```python
from build123d import *

# Parameters (mm, degrees)
F0_W     = 214.5938575268
F0_H     = 46.5465178713
F1_DEPTH = 25.4


with BuildPart() as f1:
    # F0 (on Front) → F1 (new body)
    with BuildSketch(Plane.XZ):
        with Locations((39.4191890955, 25.6276843138)):
            Rectangle(F0_W, F0_H)
        Polygon((-39.0857293959, 9.3650380149), (-58.7409636363, 9.3650380149), (-58.7409636363, 44.6240742319), (-54.6432292894, 44.6240742319), (-54.6432292894, 13.0769216701), (-39.0857293959, 13.0769216701), align=None, mode=Mode.SUBTRACT)
        Polygon((-6.697422326, 9.3650380149), (-10.9417799358, 9.3650380149), (-15.3327608085, 20.5778591187), (-29.4626131423, 20.5778591187), (-33.7995749182, 9.3650380149), (-37.951328362, 9.3650380149), (-24.0144013741, 44.7706974947), (-20.5648961894, 44.7706974947), align=None, mode=Mode.SUBTRACT)
        with BuildLine():
            Line((25.6908847439, 44.6240742319), (25.6908847439, 9.3650380149))
            Line((25.6908847439, 9.3650380149), (21.0143743593, 9.3650380149))
            Line((21.0143743593, 9.3650380149), (1.7449908106, 38.9520690624))
            Line((1.7449908106, 38.9520690624), (1.5520654647, 38.9520690624))
            add(Edge.make_bspline(
                [(1.5520654647, 38.9520690624), (1.9379161565, 33.743084723), (1.9379161565, 29.4061229472)],
                knots=[0, 0, 0, 1, 1, 1], degree=2))
            Line((1.9379161565, 29.4061229472), (1.9379161565, 9.3650380149))
            Line((1.9379161565, 9.3650380149), (-1.851137637, 9.3650380149))
            Line((-1.851137637, 9.3650380149), (-1.851137637, 44.6240742319))
            Line((-1.851137637, 44.6240742319), (2.7790706647, 44.6240742319))
            Line((2.7790706647, 44.6240742319), (22.0021521303, 15.152798392))
            Line((22.0021521303, 15.152798392), (22.1950774762, 15.152798392))
            add(Edge.make_bspline(
                [(22.1950774762, 15.152798392), (22.1487753932, 15.8010275542), (21.9790010888, 19.3354198911)],
                knots=[0, 0, 0, 1, 1, 1], degree=2))
            add(Edge.make_bspline(
                [(21.9790010888, 19.3354198911), (21.8092267844, 22.869812228), (21.8555288674, 24.3900639537)],
                knots=[0, 0, 0, 1, 1, 1], degree=2))
            Line((21.8555288674, 24.3900639537), (21.8555288674, 44.6240742319))
            Line((21.8555288674, 44.6240742319), (25.6908847439, 44.6240742319))
        make_face(mode=Mode.SUBTRACT)
        with BuildLine():
            add(Edge.make_bspline(
                [(58.9705069119, 40.0671775617), (63.5274035821, 35.5102808915), (63.5274035821, 27.3302462253)],
                knots=[0, 0, 0, 1, 1, 1], degree=2))
            add(Edge.make_bspline(
                [(63.5274035821, 27.3302462253), (63.5274035821, 18.6023035767), (58.7891570867, 13.9836707958)],
                knots=[0, 0, 0, 1, 1, 1], degree=2))
            add(Edge.make_bspline(
                [(58.7891570867, 13.9836707958), (54.0509105914, 9.3650380149), (45.1531936384, 9.3650380149)],
                knots=[0, 0, 0, 1, 1, 1], degree=2))
            Line((45.1531936384, 9.3650380149), (35.383454122, 9.3650380149))
            Line((35.383454122, 9.3650380149), (35.383454122, 44.6240742319))
            Line((35.383454122, 44.6240742319), (46.1872734925, 44.6240742319))
            add(Edge.make_bspline(
                [(46.1872734925, 44.6240742319), (54.4136102417, 44.6240742319), (58.9705069119, 40.0671775617)],
                knots=[0, 0, 0, 1, 1, 1], degree=2))
        make_face(mode=Mode.SUBTRACT)
        with BuildLine():
            add(Edge.make_bspline(
                [(97.7292089034, 40.3565655805), (101.9967175548, 35.533431933), (101.9967175548, 27.0447167133)],
                knots=[0, 0, 0, 1, 1, 1], degree=2))
            add(Edge.make_bspline(
                [(101.9967175548, 27.0447167133), (101.9967175548, 18.5791525352), (97.7137748758, 13.7290093392)],
                knots=[0, 0, 0, 1, 1, 1], degree=2))
            add(Edge.make_bspline(
                [(97.7137748758, 13.7290093392), (93.4308321967, 8.8788661433), (85.8141395406, 8.8788661433)],
                knots=[0, 0, 0, 1, 1, 1], degree=2))
            add(Edge.make_bspline(
                [(85.8141395406, 8.8788661433), (78.02767258, 8.8788661433), (73.7948904909, 13.644122187)],
                knots=[0, 0, 0, 1, 1, 1], degree=2))
            add(Edge.make_bspline(
                [(73.7948904909, 13.644122187), (69.5621084018, 18.4093782308), (69.5621084018, 27.0910187964)],
                knots=[0, 0, 0, 1, 1, 1], degree=2))
            add(Edge.make_bspline(
                [(69.5621084018, 27.0910187964), (69.5621084018, 35.7032062374), (73.8064660117, 40.4414527327)],
                knots=[0, 0, 0, 1, 1, 1], degree=2))
            add(Edge.make_bspline(
                [(73.8064660117, 40.4414527327), (78.0508236215, 45.1796992281), (85.8604416236, 45.1796992281)],
                knots=[0, 0, 0, 1, 1, 1], degree=2))
            add(Edge.make_bspline(
                [(85.8604416236, 45.1796992281), (93.4617002521, 45.1796992281), (97.7292089034, 40.3565655805)],
                knots=[0, 0, 0, 1, 1, 1], degree=2))
        make_face(mode=Mode.SUBTRACT)
        with BuildLine():
            Line((137.3946600207, 44.6240742319), (137.3946600207, 9.3650380149))
            Line((137.3946600207, 9.3650380149), (132.7181496361, 9.3650380149))
            Line((132.7181496361, 9.3650380149), (113.4487660875, 38.9520690624))
            Line((113.4487660875, 38.9520690624), (113.2558407416, 38.9520690624))
            add(Edge.make_bspline(
                [(113.2558407416, 38.9520690624), (113.6416914334, 33.743084723), (113.6416914334, 29.4061229472)],
                knots=[0, 0, 0, 1, 1, 1], degree=2))
            Line((113.6416914334, 29.4061229472), (113.6416914334, 9.3650380149))
            Line((113.6416914334, 9.3650380149), (109.8526376399, 9.3650380149))
            Line((109.8526376399, 9.3650380149), (109.8526376399, 44.6240742319))
            Line((109.8526376399, 44.6240742319), (114.4828459415, 44.6240742319))
            Line((114.4828459415, 44.6240742319), (133.7059274071, 15.152798392))
            Line((133.7059274071, 15.152798392), (133.898852753, 15.152798392))
            add(Edge.make_bspline(
                [(133.898852753, 15.152798392), (133.85255067, 15.8010275542), (133.6827763656, 19.3354198911)],
                knots=[0, 0, 0, 1, 1, 1], degree=2))
            add(Edge.make_bspline(
                [(133.6827763656, 19.3354198911), (133.5130020612, 22.869812228), (133.5593041442, 24.3900639537)],
                knots=[0, 0, 0, 1, 1, 1], degree=2))
            Line((133.5593041442, 24.3900639537), (133.5593041442, 44.6240742319))
            Line((133.5593041442, 44.6240742319), (137.3946600207, 44.6240742319))
        make_face(mode=Mode.SUBTRACT)
    extrude(amount=F1_DEPTH)


solid = f1.part
```
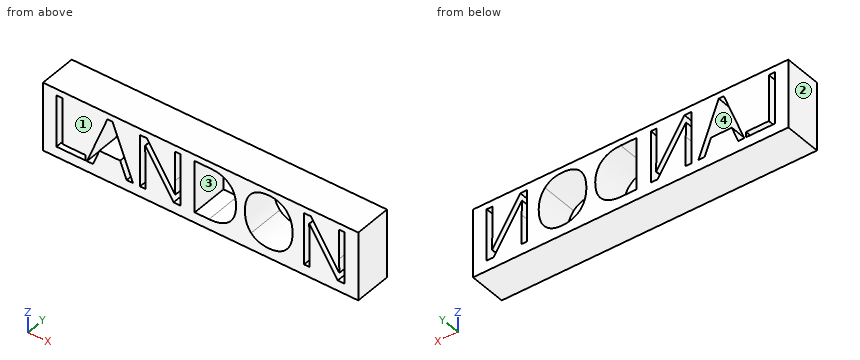
The listing builds one solid part. Answer for the finished solid, in the listing's coordinates (mm). Face numbers are marked on the shaded views. Give positions to 0.01 mm unless a question says otherwise; leave off trailing zeros. Order: outer loops, then holes, each group sorted by start corner. A loop starts at its lowest first (then second) coordinate and runs counter-clockwise, first axis right, second up. Notation, with made-up numbers: (0, 63) -> (20, 63) arc R28 cw to (20, 90) -> close; hole circle Ø9 at (4, -9.5). An arc over 180 degrees is marked (long way). Write each question's results on one line, items separated by ' | '.
Q1. The part is cut by section A-A, the plane x = 7.5. Give the vertices of the cut face in (y, z).
Checked values:
outline: (-25.4, 2.35) -> (0, 2.35) -> (0, 30.12) -> (-25.4, 30.12) -> close; (-25.4, 37.39) -> (0, 37.39) -> (0, 48.9) -> (-25.4, 48.9) -> close
Q2. The part is cut by section B-B, the plane y = -7.75. State how many separate pieces and enclosed holes the cut face has, and give its area (3 significant figures).
Checked values:
separate pieces: 1 | enclosed holes: 6 | area: 6,710 mm^2
Q3. Determine the mould class of the marked faces 1, 2, 3 and 4 for opening direction X: pulls with the +X half, pulls with the -X half, needs draft (parallel to the pull), parting line crosses it, or undercut.
Checked values:
face 1: needs draft | face 2: pulls with the -X half | face 3: undercut | face 4: undercut
Q4. Straight lines are drawn through the part: probe 1 along Z at (x, y) = (1, -6.25); probe 2 along Z at (x, y) = (-50, -7.25). For each, find the intervals that lie inside material, in ascending order. Write a range as from..to.
Checked values:
probe 1: z = 2.35..9.37, 44.62..48.9 | probe 2: z = 2.35..9.37, 13.08..48.9
